Autodesk Inventor part; units mm, degrees
ref_plane "YZ Plane" through (0, 0, 0) normal (1, 0, 0) x (0, 1, 0)
ref_plane "XZ Plane" through (0, 0, 0) normal (0, 1, 0) x (-1, 0, 0)
ref_plane "XY Plane" through (0, 0, 0) normal (0, 0, 1) x (1, 0, 0)
ref_plane "Work Plane1" through (0, 0, 0) normal (0, 0, 1) x (1, 0, 0)
sketch "Sketch1" plane through (0, 0, 0) normal (0, 0, 1) x (1, 0, 0)
  line L0 (-42, -2) -> (-73.5901, -2)
  arc A0 (-39.1716, -4) -> (-42, -2) centre (-42, -5) ccw
  arc A1 (-39.1716, -4) -> (-36.3431, -6) centre (-36.3431, -3) ccw
  line L1 (-36, -6) -> (-36.3431, -6)
  arc A2 (-36, -6) -> (-33.1612, -3.9702) centre (-36, -3) ccw
  line L2 (-33, -2.5071) -> (-33, -2)
  line L3 (-32, -1) -> (0, -1)
  line L4 (0, 0) -> (0, -1)
  line L5 (-83.8327, 0) -> (0, 0)
  line L6 (-83.8327, 0) -> (-83.8327, -6)
  line L7 (-77.8327, -6) -> (-83.8327, -6)
  line L8 (-41.75, -176) -> (-73.5901, -176)
  line L9 (-77.8327, -172) -> (-83.8327, -172)
  line L10 (-83.8327, -178) -> (-83.8327, -172)
  line L11 (-83.8327, -178) -> (0, -178)
  line L12 (0, -178) -> (0, -177)
  line L13 (-31.75, -177) -> (0, -177)
  line L14 (-32.75, -175) -> (-32.75, -176)
  arc A3 (-32.75, -175) -> (-35.75, -172) centre (-35.75, -175) ccw
  line L15 (-35.75, -172) -> (-36.0931, -172)
  arc A4 (-36.0931, -172) -> (-38.9216, -174) centre (-36.0931, -175) ccw
  arc A5 (-41.75, -176) -> (-38.9216, -174) centre (-41.75, -173) ccw
  line L16 (0, 0) -> (-83.8327, 0)
  line L17 (-83.8327, 0) -> (-83.8327, -178)
  line L18 (-83.8327, -178) -> (0, -178)
  line L19 (0, -178) -> (0, 0)
  circle A6 centre (9.325, -58.5) radius 3
  line L20 (-30.35, -55) -> (-30.35, -62)
  line L21 (-30.35, -62) -> (50, -62)
  line L22 (50, -62) -> (50, -55)
  line L23 (50, -55) -> (-30.35, -55)
  circle A7 centre (-81.3327, -118.5) radius 1.75
  line L24 (50, -123) -> (-83.8327, -123)
  line L25 (50, -116) -> (50, -123)
  line L26 (-30.55, -116) -> (50, -116)
  line L27 (-30.55, -116) -> (-30.55, -121)
  line L28 (-30.55, -121) -> (-46.95, -121)
  line L29 (-46.95, -121) -> (-46.95, -116)
  line L30 (-83.8327, -116) -> (-46.95, -116)
  line L31 (-83.8327, -123) -> (-83.8327, -116)
  circle A8 centre (9.325, -119.5) radius 3
  line L32 (0, -55) -> (50, -55)
  line L33 (50, -55) -> (50, -123)
  line L34 (50, -123) -> (0, -123)
  line L35 (0, -123) -> (0, -55)
  arc A9 (-32, -1) -> (-33, -2) centre (-32, -2) ccw
  circle A10 centre (-80.8327, -3) radius 2.3
  arc A11 (-73.5901, -2) -> (-77.8327, -6) centre (-73.5901, -6.25) ccw
  arc A12 (-33, -2.5071) -> (-33.1612, -3.9702) centre (-35.2466, -3) ccw
  arc A13 (-32.75, -176) -> (-31.75, -177) centre (-31.75, -176) ccw
  circle A14 centre (-35.2466, -175) radius 2.3
  circle A15 centre (-80.8327, -175) radius 2.3
  arc A16 (-77.8327, -172) -> (-73.5901, -176) centre (-73.5901, -171.75) ccw
  point P0 (0, -123)
extrude "Extrusion1" add sketch "Sketch1" along normal blind 1 contours A0 A1 L1 A2 A12 L2 A9 L3 L19 L23 L20 L21 L26 L27 L28 L29 L30 L17 L7 A11 L0 | L0 A11 L7 L6 L5 L4 L3 A9 L2 A12 A2 L1 A1 A0 | L30 L29 L28 L27 L26 L19 L24 L17 | L24 L19 L13 A13 L14 A3 L15 A4 A5 L8 A16 L9 L17 | L9 A16 L8 A5 A4 L15 A3 L14 A13 L13 L12 L11 L10 | L19 L26 L25 L24 | L23 L22 L21 L19 | L19 L21 L20 L23 | L19 L21 L33 L26 | A6 | A7 | A8 | A10 | A14 | A15
sketch "Sketch3" plane through (0, 0, 1) normal (0, 0, 1) x (1, 0, 0)
  circle A0 centre (-81.3327, -59.5) radius 1.75
  circle A1 centre (-81.3327, -118.5) radius 1.75
  circle A2 centre (-77.3327, -3) radius 2.3
  circle A3 centre (-35.2466, -3) radius 2.3
  circle A4 centre (-35.2466, -175) radius 2.3
  circle A5 centre (-77.3327, -175) radius 2.3
  point P0 (0, 0)
hole "Hole1" at (-35.2466, -3, 1) at (-77.3327, -3, 1) at (-77.3327, -175, 1) at (-35.2466, -175, 1) direction (0, 0, -1) diameter 3.6 end through all countersink diameter 6 countersink angle 90
sketch "Sketch4" plane through (0, 0, 1) normal (0, 0, 1) x (1, 0, 0)
  circle A0 centre (-81.3327, -59.5) radius 1.75
  circle A1 centre (-81.3327, -118.5) radius 1.75
  point P0 (0, 0)
hole "Hole2" at (-81.3327, -59.5, 1) at (-81.3327, -118.5, 1) direction (0, 0, -1) diameter 3.1 end through all countersink diameter 5 countersink angle 90
sketch "Sketch5" plane through (0, 0, 1) normal (0, 0, 1) x (1, 0, 0)
  line L0 (-54.55, -139.6) -> (-54.55, -129.1)
  line L1 (-44.05, -129.1) -> (-54.55, -129.1)
  line L2 (-44.05, -129.1) -> (-44.05, -139.6)
  line L3 (-54.55, -139.6) -> (-44.05, -139.6)
  line L4 (-76.05, -140.6) -> (-76.05, -129.6)
  line L5 (-76.05, -129.6) -> (-63.05, -129.6)
  line L6 (-63.05, -129.6) -> (-63.05, -140.6)
  line L7 (-63.05, -140.6) -> (-76.05, -140.6)
  line L8 (-77.05, -123) -> (-77.05, -141.6)
  line L9 (-77.05, -141.6) -> (-35.75, -141.6)
  line L10 (-35.75, -141.6) -> (-35.75, -123)
  line L11 (-35.75, -123) -> (-77.05, -123)
  circle A0 centre (-73.6, -126.3) radius 1.5
  circle A1 centre (-39.2, -126.3) radius 1.5
  line L12 (-68.4939, -42.5) -> (-68.4939, -56.8)
  line L13 (-48.1, -42.4061) -> (-68.4, -42.4061)
  line L14 (-47.9, -56.9) -> (-47.9, -42.4)
  line L15 (-68.4, -56.8939) -> (-48.1, -56.8939)
  line L16 (-68.8327, -42) -> (-68.8327, -57)
  line L17 (-83.8327, -42) -> (-68.8327, -42)
  line L18 (-83.8327, -57) -> (-83.8327, -42)
  line L19 (-68.8327, -57) -> (-83.8327, -57)
  line L20 (-46.9, -41) -> (-83.8327, -41)
  line L21 (-83.8327, -41) -> (-83.8327, -57)
  line L22 (-83.8327, -57) -> (-46.9, -57)
  line L23 (-46.9, -57) -> (-46.9, -41)
  line L24 (50, -123) -> (50, -55)
  line L25 (50, -55) -> (0, -55)
  line L26 (0, -55) -> (0, 0)
  line L27 (0, 0) -> (-35.2466, 0)
  circle A2 centre (-35.2466, -3) radius 3
  line L28 (-35.2466, 0) -> (-77.3327, 0)
  circle A3 centre (-77.3327, -3) radius 3
  line L29 (-77.3327, 0) -> (-83.8327, 0)
  line L30 (-83.8327, 0) -> (-83.8327, -59.5)
  circle A4 centre (-81.3327, -59.5) radius 2.5
  line L31 (-83.8327, -59.5) -> (-83.8327, -118.5)
  circle A5 centre (-81.3327, -118.5) radius 2.5
  line L32 (-83.8327, -118.5) -> (-83.8327, -178)
  line L33 (-83.8327, -178) -> (-77.3327, -178)
  circle A6 centre (-77.3327, -175) radius 3
  line L34 (-77.3327, -178) -> (-35.2466, -178)
  circle A7 centre (-35.2466, -175) radius 3
  line L35 (-35.2466, -178) -> (0, -178)
  line L36 (0, -178) -> (0, -123)
  line L37 (0, -123) -> (50, -123)
  line L38 (-43.05, -140.6) -> (-43.05, -128.1)
  line L39 (-43.05, -128.1) -> (-55.55, -128.1)
  line L40 (-55.55, -128.1) -> (-55.55, -140.6)
  line L41 (-55.55, -140.6) -> (-43.05, -140.6)
  line L42 (-62.05, -141.6) -> (-62.05, -128.6)
  line L43 (-62.05, -128.6) -> (-77.05, -128.6)
  line L44 (-77.05, -128.6) -> (-77.05, -141.6)
  line L45 (-77.05, -141.6) -> (-62.05, -141.6)
  line L46 (-30, -4.4) -> (-2, -4.4)
  line L47 (-2, -173.6) -> (-30, -173.6)
  line L48 (-2, -4.4) -> (-29.4, -4.4)
  line L49 (-29.4, -4.4) -> (-29.4, -2.4)
  line L50 (-29.4, -2.4) -> (-2, -2.4)
  line L51 (-2, -2.4) -> (-2, -4.4)
  line L52 (-2, -173.6) -> (-29.4, -173.6)
  line L53 (-29.4, -173.6) -> (-29.4, -175.6)
  line L54 (-29.4, -175.6) -> (-2, -175.6)
  line L55 (-2, -175.6) -> (-2, -173.6)
  line L56 (-30, -51) -> (-2, -51)
  line L57 (-30, -4.4) -> (-2, -4.4)
  line L58 (50, -123) -> (50, -55)
  line L59 (50, -89) -> (-83.8327, -89) construction
  line L60 (-83.8327, 0) -> (-83.8327, -178)
  line L61 (-2, -51) -> (-29.4, -51)
  line L62 (-29.4, -51) -> (-29.4, -2.4)
  line L63 (-29.4, -2.4) -> (-2, -2.4)
  line L64 (-2, -2.4) -> (-2, -51)
  line L65 (-30, -127) -> (-2, -127)
  line L66 (-30, -173.6) -> (-2, -173.6)
  line L67 (-29.4, -127) -> (-29.4, -175.6)
  line L68 (-29.4, -175.6) -> (-2, -175.6)
  line L69 (-2, -175.6) -> (-2, -127)
  point P0 (-29.4, -4.4)
  point P1 (-29.4, -127)
  point P2 (-2, -173.6)
  point P3 (-2, -4.4)
  point P4 (-29.4, -4.4)
  point P5 (-29.4, -51)
  dimension "d16" = 1
  dimension "d17" = 0
  dimension "d18" = 0
  dimension "d19" = 1
  dimension "d20" = 1
  dimension "d21" = 1
  dimension "d28" = 2
  dimension "d29" = 2
extrude "Extrusion2" cut sketch "Sketch5" against normal up to next contours L0 L1 L2 L3 | L4 L5 L6 L7 | L43 L42 L9 L8 | L17 L21 L20 L23 L22 L16 | L16 L19 L18 L17 | L41 L40 L39 L38 | L49 L50 L51 L46 | L46 L64 L56 L62 | L55 L54 L53 L47 | L47 L67 L65 L69
fillet "Fillet1" radius 5 8 edges at (-2, -2.4, 0.5) (-2, -51, 0.5) (-29.4, -51, 0.5) (-29.4, -2.4, 0.5) (-29.4, -127, 0.5) (-2, -175.6, 0.5) (-2, -127, 0.5) (-29.4, -175.6, 0.5)
properties part number "ceil" material "ABS Plastic"
Can you work these out from the model? Positions are in its coordinate system, mm. A direction names the side the tool comes from. Give positions to 0.01 mm unless a question says otherwise; leave off trailing zeros. Order: outer loops, then holes, each group sorted by start corner. A loop starts at its lowest first (then second) coordinate and runs counter-clockwise, first axis right, second up. Notation, with made-up numbers: M 11,-0.75 L 24,-0.75 A14 cw 24,26.25 Z; hole C -25,80 d2. An arc over 180 degrees is marked long. One line per item, written item: value.
1) On a 3-axis mill with a long thin cutter (end or side, diameter ignored), from which of +Z, -Z, +X, -X, +Y, -Y can I reach the whole of each face in a straight line? I mean faces 4 (the face through (-33, -88, 1)), 5 (the face through (-3.5, -128.43, 0.49)). Say none if no direction works.
Answer sheet:
face 4: +Z, +X, -X, +Y, -Y
face 5: +Z, -Z
2) Please list where these lines run through material, in increasing order: line 1 along Y through (x, z) = (-23.5, 0.8); line 2 along Y through (x, z) = (-54, 0.7); line 3 along X through (y, z) = (-8, 0.6).
Answer sheet:
line 1: y = -178 to -175.6, -127 to -51, -2.4 to 0
line 2: y = -178 to -140.6, -128.1 to -57, -41 to 0
line 3: x = -83.83 to -29.4, -2 to 0
3) I want a section at B-B, the plane y = -161. List the corners of the cut face in (x, z) for me, plus the area to 3 significant figures.
Answer sheet:
outline: M -83.83,0 L -29.4,0 L -29.4,1 L -83.83,1 Z; M -2,0 L 0,0 L 0,1 L -2,1 Z
area: 56.4 mm^2
4) For P1, Ø0.5, axis at y = -37, z = 0.5, coming from the +X side; P2, Ø0.5, axis at x = -19, z = 0.5, coming from the +Y side, each with a flat end and sliding along its axis, tell me the tip position at first contact or that it passes through.
Answer sheet:
P1: stops at x = 0
P2: stops at y = 0
5) I want a section at D-D, the plane z = 0.65. Count the separate pieces of the cut face and the enclosed holes in it, plus the area to 3 significant figures.
Answer sheet:
separate pieces: 1
enclosed holes: 10
area: 14,600 mm^2
6) I want a section at A-A, the plane x = -72.5. List the corners of the cut face in (y, z) for me.
Answer sheet:
outline: M -178,0 L -141.6,0 L -141.6,1 L -178,1 Z; M -128.6,0 L -57,0 L -57,1 L -128.6,1 Z; M -41,0 L 0,0 L 0,1 L -41,1 Z
7) I want a section at C-C, the plane x = -12. List the corners of the cut face in (y, z) for me, plus the area to 3 significant figures.
Answer sheet:
outline: M -178,0 L -175.6,0 L -175.6,1 L -178,1 Z; M -127,0 L -51,0 L -51,1 L -127,1 Z; M -2.4,0 L 0,0 L 0,1 L -2.4,1 Z
area: 80.8 mm^2
8) We'd pull the mould along X, two halves only. Please class faces 1 (the face through (-33, -88, 0)), 2 (the face through (-27.9, -49.57, 0.49)), 3 (the face through (-27.97, -128.5, 0.49)): released by +X, released by -X, zero draft, split by the parting line, or undercut.
Answer sheet:
face 1: zero draft
face 2: undercut
face 3: undercut
